Verification items for the finished model (mm, model axes). Face numbers are marked on the shaded views. A direction names the side the tool comes from. Round coordinates to 2 decimals unless told otherwise and drop trailing zeros. Loops run counter-clockwise (first coordinate to the right, second up) from the corner with the lowest first, then second, coordinate; pieces in that order, holes last. Notation, with made-up numbers: (78.25, 77) - (121.25, 77) arc R5 ccw to (121.25, 85) - close; hole circle Ø2 at (0, 24). An arc over 180 degrees is marked (long way). Use a Markdown table: item, result. Add a question column.
Autodesk Inventor part; units mm, degrees
ref_plane "YZ Plane" through (0, 0, 0) normal (1, 0, 0) x (0, 1, 0)
ref_plane "XZ Plane" through (0, 0, 0) normal (0, 1, 0) x (-1, 0, 0)
ref_plane "XY Plane" through (0, 0, 0) normal (0, 0, 1) x (1, 0, 0)
sketch "Sketch1" plane through (0, 0, 0) normal (0, 0, 1) x (1, 0, 0)
  line L0 (-11.25, 59.5) -> (-8.75, 59.5) construction
  line L1 (-8.75, 59.5) -> (-8.75, 57) construction
  line L2 (-8.75, 57) -> (-11.25, 57) construction
  line L3 (-11.25, 57) -> (-11.25, 59.5) construction
  line L4 (0, 59.5) -> (-11.25, 59.5) construction
  circle A0 centre (-8.75, 57) radius 1.5
  line L5 (-8.75, 57) -> (-2.5, 57) construction
  line L6 (-2.5, 57) -> (-2.5, 34.5) construction
  line L7 (-2.5, 34.5) -> (-8.75, 34.5) construction
  line L8 (-8.75, 34.5) -> (-8.75, 57) construction
  circle A1 centre (-8.75, 34.5) radius 1.5
  circle A2 centre (-2.5, 34.5) radius 1.5
  circle A3 centre (-2.5, 57) radius 1.5
  line L9 (-11.25, 59.5) -> (0, 59.5)
  line L10 (0, 59.5) -> (0, 2)
  line L11 (0, 2) -> (-11.25, 2)
  line L12 (-11.25, 2) -> (-11.25, 59.5)
  line L13 (-9.95, 40.4) -> (0, 40.4) construction
  line L14 (-1.3, 40.4) -> (0, 40.4) construction
  line L15 (-9.95, 37) -> (0, 37) construction
  line L16 (-9.95, 40.4) -> (-1.3, 40.4)
  line L17 (-1.3, 40.4) -> (-1.3, 37)
  line L18 (-1.3, 37) -> (-9.95, 37)
  line L19 (-9.95, 37) -> (-9.95, 40.4)
  line L20 (0, 59.5) -> (-1.3, 59.5) construction
  line L21 (-1.3, 59.5) -> (-1.3, 40.4) construction
  line L22 (-1.3, 40.4) -> (0, 40.4) construction
  line L23 (0, 40.4) -> (0, 59.5) construction
  line L24 (0, 59.5) -> (-9.95, 59.5) construction
  line L25 (-9.95, 59.5) -> (-9.95, 37) construction
  line L26 (-9.95, 37) -> (0, 37) construction
  line L27 (0, 37) -> (0, 59.5) construction
  point P0 (0, 0)
  dimension "d0" = 2.5
  dimension "d1" = 2.5
  dimension "d2" = 3
  dimension "d3" = 6.25
  dimension "d4" = 22.5
  dimension "d5" = 3
  dimension "d6" = 3
  dimension "d7" = 3
  dimension "d8" = 11.25
  dimension "d9" = 57.5
  dimension "d10" = 9.95
  dimension "d11" = 1.3
extrude "Extrusion1" add sketch "Sketch1" along normal blind 2
sketch "Sketch2" plane through (0, 2, 0) normal (1, 0, 0) x (0, 0, -1)
  line L0 (0, 0) -> (0, 57.5) construction
  line L1 (0, 0) -> (18, 0) construction
  line L2 (18, 0) -> (18, -30) construction
  line L3 (18, 0) -> (48, 0) construction
  line L4 (18, -30) -> (18, -17) construction
  point P0 (0, -2)
  dimension "d14" = 18
  dimension "d15" = 30
  dimension "d16" = 90
  dimension "d17" = 13
sketch "Sketch7" plane through (0, 0, 0) normal (0, 0, -1) x (-1, 0, 0)
  line L0 (1.4108, -1.2142) -> (2.825, -2.6284)
  line L1 (2.825, 0.2) -> (1.4108, -1.2142)
  line L2 (2.825, 0.2) -> (2.825, 2)
  line L3 (5.625, 0.2) -> (5.625, 2) construction
  line L4 (2.825, -2.6284) -> (5.625, -2.6284)
  line L5 (5.625, 2) -> (5.625, -3) construction
  line L6 (8.425, -2.6284) -> (5.625, -2.6284)
  line L7 (8.425, 0.2) -> (5.625, 0.2) construction
  line L8 (8.425, 2) -> (8.425, 0.2) construction
  line L9 (8.425, 2) -> (8.425, 0.2)
  line L10 (8.425, 0.2) -> (9.8392, -1.2142)
  line L11 (9.8392, -1.2142) -> (8.425, -2.6284)
  line L12 (8.425, 0.2) -> (10.425, 0.2) construction
  line L13 (9.95, 37) -> (1.3, 37)
  line L14 (1.3, 37) -> (1.3, 40.4)
  line L15 (1.3, 40.4) -> (9.95, 40.4)
  line L16 (9.95, 40.4) -> (9.95, 37)
  circle A0 centre (2.5, 57) radius 1.5
  circle A1 centre (8.75, 57) radius 1.5
  circle A2 centre (2.5, 34.5) radius 1.5
  circle A3 centre (8.75, 34.5) radius 1.5
  line L17 (11.25, 59.5) -> (0, 59.5)
  line L18 (0, 59.5) -> (0, 2)
  line L19 (0, 2) -> (11.25, 2)
  line L20 (11.25, 2) -> (11.25, 59.5)
  line L21 (11.25, 2) -> (0, 2) construction
  line L22 (5.625, 2) -> (5.625, 3.9478) construction
  line L23 (2.825, 2) -> (8.425, 2)
  line L24 (2.825, 2) -> (8.425, 2)
  line L25 (8.425, 2) -> (8.425, 0.2)
  line L26 (8.425, 0.2) -> (2.825, 0.2)
  line L27 (2.825, 0.2) -> (2.825, 2)
  line L28 (0, 2) -> (11.25, 2)
  line L29 (11.25, 2) -> (11.25, 4)
  line L30 (11.25, 4) -> (0, 4)
  line L31 (0, 4) -> (0, 2)
  dimension "d24" = 5
  dimension "d25" = 2.8
  dimension "d26" = 1.8
  dimension "d28" = 1.8
  dimension "d29" = 2
  dimension "d30" = 45
  dimension "d31" = 2
  dimension "d37" = 2
extrude "Extrusion2" add sketch "Sketch7" against normal blind 20 contours L1 L26 L10 L11 L6 L4 L0 | L2 L19 L9 L26 | L19 L18 L30 L20
fillet "Fillet1" radius 10 1 edges at (-5.625, 4, 2)
properties part number "prox_base"
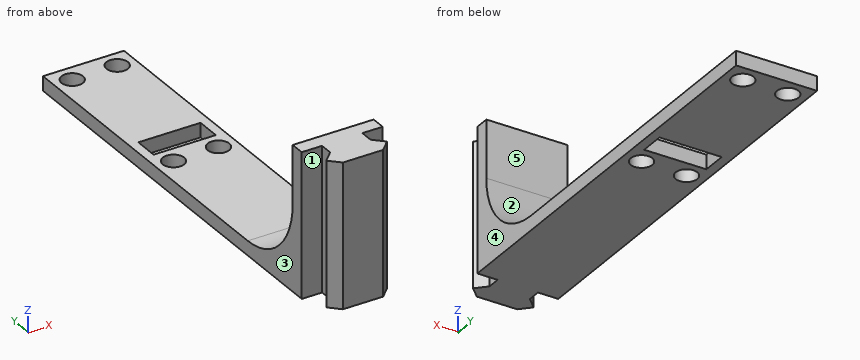
Q1. Section check A-A on x = -6.5. Record the cut outline in (y, z).
Q2. Set-up check for the marked faces 4 and 5: record each of +Z, -Z, +X, -X, +Y, -Y from which the full face is reachable in a straight line by a thin tool's end or side.
Q3. Section check C-C on z = 15.75. Record the cut outline in (x, y) (3 decimals).
Q4. Section check D-D on x = -2.25. Record the cut outline in (y, z) (3 decimals).
Q5. Go/stop test with flat-tipped pins: pin 1 Ø4 at (x, y) = (-2.5, 34.5) entering from +Z; pin 2 Ø1.5 at (x, z) = (-8.5, 17) entering from +Y; pin 3 Ø0.9 at (y, z) = (1.5, 5) entering from -X (3 decimals). Record where each tip stops, or that it passes through.
Q6. Thickness scan on line 1 along Y through (x, z) = (-4.5, 1.25); line 2 along Y through (x, z) = (-8.75, 1.5) (3 decimals); line 3 along Y through (x, z) = (-7, 14.75). Record the ranges inside material, lowest first.
Q7. Release check for a two-part mould opening along Y. For the marked faces 1, 2 and 3 record: +Y half, -Y half, draft (parallel to the pull), parting line (faces both ways), or undercut.
Q8. Section check B-B on y = 57. Record the cut outline in (x, z), plus the area to 3 significant figures.
Determined:
| question | item | result |
|---|---|---|
| 1 | outline | (-2.63, 0) - (37, 0) - (37, 2) - (14, 2) arc R10 cw to (4, 12) - (4, 20) - (-2.63, 20) - close; (40.4, 0) - (59.5, 0) - (59.5, 2) - (40.4, 2) - close |
| 2 | face 4 | +Z, -Z, +X, +Y, -Y |
| 2 | face 5 | +Z, +X, -X, +Y |
| 3 | outline | (-11.25, 2) - (-8.425, 2) - (-8.425, 0.2) - (-9.839, -1.214) - (-8.425, -2.628) - (-2.825, -2.628) - (-1.411, -1.214) - (-2.825, 0.2) - (-2.825, 2) - (0, 2) - (0, 4) - (-11.25, 4) - close |
| 4 | outline | (-2.053, 0) - (-0.375, 0) - (-0.375, 20) - (-2.053, 20) - close; (2, 0) - (33.021, 0) - (33.021, 2) - (14, 2) arc R10 cw to (4, 12) - (4, 20) - (2, 20) - close; (35.979, 0) - (37, 0) - (37, 2) - (35.979, 2) - close; (40.4, 0) - (55.521, 0) - (55.521, 2) - (40.4, 2) - close; (58.479, 0) - (59.5, 0) - (59.5, 2) - (58.479, 2) - close |
| 5 | pin 1 | stops at z = 2 |
| 5 | pin 2 | stops at y = 4 |
| 5 | pin 3 | stops at x = -8.425 |
| 6 | line 1 | y = -2.63 to 37, 40.4 to 59.5 |
| 6 | line 2 | y = -2.303 to -0.125, 2 to 33, 36 to 37, 40.4 to 55.5, 58.5 to 59.5 |
| 6 | line 3 | y = -2.63 to 4 |
| 7 | face 1 | undercut |
| 7 | face 2 | +Y half |
| 7 | face 3 | draft |
| 8 | outline | (-11.25, 0) - (-10.25, 0) - (-10.25, 2) - (-11.25, 2) - close; (-7.25, 0) - (-4, 0) - (-4, 2) - (-7.25, 2) - close; (-1, 0) - (0, 0) - (0, 2) - (-1, 2) - close |
| 8 | area | 10.5 mm² |
